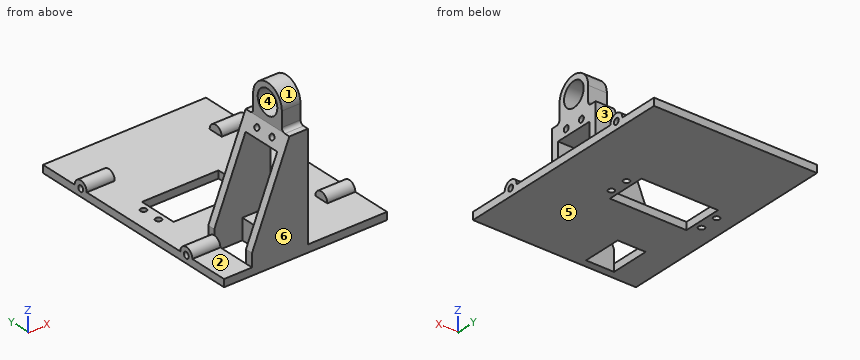
Autodesk Inventor part; units mm, degrees
ref_plane "YZ Plane" through (0, 0, 0) normal (1, 0, 0) x (0, 1, 0)
ref_plane "XZ Plane" through (0, 0, 0) normal (0, 1, 0) x (-1, 0, 0)
ref_plane "XY Plane" through (0, 0, 0) normal (0, 0, 1) x (1, 0, 0)
sketch "Sketch1" plane through (0, 0, 0) normal (0, 0, 1) x (1, 0, 0)
  line L0 (-30.65, -10.5) -> (10.35, -10.5)
  line L1 (10.35, -10.5) -> (10.35, 10.5)
  line L2 (10.35, 10.5) -> (-30.65, 10.5)
  line L3 (-30.65, 10.5) -> (-30.65, -10.5)
  line L4 (-30.65, -10.5) -> (10.35, 10.5) construction
  line L5 (10.35, -10.5) -> (-30.65, 10.5) construction
  line L6 (-43.65, -60) -> (43.65, -60)
  line L7 (43.65, -60) -> (43.65, 60)
  line L8 (43.65, 60) -> (-43.65, 60)
  line L9 (-43.65, 60) -> (-43.65, -60)
  line L10 (-43.65, -60) -> (43.65, 60) construction
  line L11 (43.65, -60) -> (-43.65, 60) construction
  point P0 (-10.15, 0)
  point P1 (0, 0)
  point P2 (-10.15, 0)
  point P3 (0, 0)
  dimension "d0" = 41
  dimension "d1" = 21
  dimension "d2" = 87.3
  dimension "d3" = 120
  dimension "d4" = 10.15
extrude "Extrusion1" add sketch "Sketch1" along normal mid plane 4
sketch "Sketch2" plane through (0, 0, 2) normal (0, 0, 1) x (1, 0, 0)
  line L0 (14, -5) -> (-34.3, -5) construction
  line L1 (-34.3, -5) -> (-34.3, 5) construction
  line L2 (-34.3, 5) -> (14, 5) construction
  line L3 (14, 5) -> (14, -5) construction
  line L4 (14, -5) -> (-34.3, 5) construction
  line L5 (-34.3, -5) -> (14, 5) construction
  point P0 (0, 0)
  point P1 (-10.15, 0)
  point P2 (-10.15, 0)
  dimension "d7" = 48.3
  dimension "d8" = 10
  dimension "d9" = 14
hole "Hole1" at (-34.3, 5, 2) at (-34.3, -5, 2) at (14, -5, 2) at (14, 5, 2) direction (0, 0, -1) diameter 3.242 end through all
sketch "Sketch3" plane through (43.65, -60, 2) normal (1, 0, 0) x (0, 0, -1)
  line L0 (4, 120) -> (0, 120)
  line L1 (0, 0) -> (0, 120)
  line L2 (4, 0) -> (0, 0)
  line L3 (4, 120) -> (4, 0)
  line L4 (0, 0) -> (0, 120)
  arc A0 (0, 29) -> (0, 21) centre (0, 25) ccw
  arc A1 (0, 99) -> (0, 91) centre (0, 95) ccw
  line L5 (0, 95) -> (0, 25) construction
  point P0 (2, 60)
  point P1 (0, 60)
  dimension "d17" = 70
extrude "Extrusion2" add sketch "Sketch3" against normal blind 15 contours L1 A1 | A0 L1
sketch "Sketch4" plane through (43.65, -60, -2) normal (1, 0, 0) x (0, 0, -1)
  line L0 (0, 120) -> (-4, 120)
  line L1 (-4, 99) -> (-4, 120)
  arc A0 (-4, 99) -> (-4, 91) centre (-4, 95) ccw
  line L2 (-4, 29) -> (-4, 91)
  arc A1 (-4, 29) -> (-4, 21) centre (-4, 25) ccw
  line L3 (-4, 0) -> (-4, 21)
  line L4 (0, 0) -> (-4, 0)
  line L5 (0, 120) -> (0, 0)
  point P0 (-2, 60)
hole "Hole2" at (43.65, 35, 2) at (43.65, -35, 2) direction (-1, 0, 0) diameter 3.242 depth 11.8 tip angle 118
mirror "Mirror1" about plane through (0, 0, 0) normal (1, 0, 0) of "Extrusion2", "Hole2"
sketch "Sketch5" plane through (0, 0, 2) normal (0, 0, 1) x (1, 0, 0)
  circle A0 centre (14, -5) radius 1.621
  circle A1 centre (-34.3, 5) radius 1.621
  circle A2 centre (-34.3, -5) radius 1.621
  circle A3 centre (14, 5) radius 1.621
  line L0 (-30.65, -10.5) -> (-30.65, 10.5)
  line L1 (-30.65, 10.5) -> (10.35, 10.5)
  line L2 (10.35, 10.5) -> (10.35, -10.5)
  line L3 (10.35, -10.5) -> (-30.65, -10.5)
  line L4 (-43.65, -31) -> (-28.65, -31)
  line L5 (-28.65, -31) -> (-28.65, -39)
  line L6 (-28.65, -39) -> (-43.65, -39)
  line L7 (-43.65, -39) -> (-43.65, -60)
  line L8 (-43.65, -60) -> (43.65, -60)
  line L9 (43.65, -60) -> (43.65, -39)
  line L10 (43.65, -39) -> (28.65, -39)
  line L11 (28.65, -39) -> (28.65, -31)
  line L12 (28.65, -31) -> (43.65, -31)
  line L13 (43.65, -31) -> (43.65, 31)
  line L14 (43.65, 31) -> (28.65, 31)
  line L15 (28.65, 31) -> (28.65, 39)
  line L16 (28.65, 39) -> (43.65, 39)
  line L17 (43.65, 39) -> (43.65, 60)
  line L18 (43.65, 60) -> (-43.65, 60)
  line L19 (-43.65, 60) -> (-43.65, 39)
  line L20 (-43.65, 39) -> (-28.65, 39)
  line L21 (-28.65, 39) -> (-28.65, 31)
  line L22 (-28.65, 31) -> (-43.65, 31)
  line L23 (-43.65, 31) -> (-43.65, -31)
  line L24 (-28.65, -35) -> (1.35, -35)
  line L25 (1.35, -35) -> (1.35, -56)
  line L26 (1.35, -56) -> (-28.65, -56)
  line L27 (-28.65, -56) -> (-28.65, -35)
  line L28 (-28.65, -31) -> (-28.65, -39)
  line L29 (10.35, 10.5) -> (10.35, -10.5)
  point P0 (0, 0)
  dimension "d27" = 45
  dimension "d28" = 4
extrude "Extrusion3" add sketch "Sketch5" along normal blind 7 contours L24 L25 L26 L27 L5
sketch "Sketch6" plane through (1.35, -56, 2) normal (1, 0, 0) x (0, 0, -1)
  line L0 (0, 21) -> (0, 0)
  line L1 (0, 21) -> (-7, 21)
  line L2 (-7, 0) -> (-7, 21)
  line L3 (0, 0) -> (-7, 0)
  line L4 (-56, -4) -> (0, -4)
  line L5 (0, -4) -> (0, 25)
  line L6 (0, 25) -> (-56, 25)
  line L7 (-56, 25) -> (-56, -4)
  line L8 (-7, 0) -> (-48, 0)
  line L9 (-48, 0) -> (-48, 21)
  line L10 (-48, 21) -> (-7, 21)
  line L11 (-7, 21) -> (-7, 0)
  line L12 (0, 25) -> (0, 87)
  line L13 (0, -4) -> (4, -4)
  point P0 (2, 56)
  point P1 (0, 10.5)
  dimension "d31" = 41
  dimension "d32" = 8
extrude "Extrusion4" add sketch "Sketch6" against normal up to surface (30 mm away) contours L0 L3 L2 L1 | L1 L10 L9 L8 L3 L5 L4 L7 L6
sketch "Sketch8" plane through (1.35, -60, 58) normal (1, 0, 0) x (0, 0, -1)
  line L0 (56, 29) -> (56, 0)
  line L1 (4.35, 9.5) -> (52.65, 9.5) construction
  line L2 (52.65, 9.5) -> (52.65, 19.5) construction
  line L3 (52.65, 19.5) -> (4.35, 19.5) construction
  line L4 (4.35, 19.5) -> (4.35, 9.5) construction
  line L5 (56, 29) -> (0, 29)
  line L6 (0, 29) -> (0, 0)
  line L7 (0, 0) -> (56, 0)
  point P0 (58, 60)
  point P1 (4.35, 14.5)
  point P2 (8, 14.5)
  point P3 (28.5, 19.5)
  point P4 (28.5, 25)
  dimension "d38" = 48.3
  dimension "d39" = 10
hole "Hole3" at (1.35, -50.5, 53.65) at (1.35, -40.5, 53.65) at (1.35, -40.5, 5.35) at (1.35, -50.5, 5.35) direction (-1, 0, 0) diameter 3.242 depth 11.8 tip angle 118
sketch "Sketch9" plane through (-43.65, -60, -2) normal (0, -1, 0) x (1, 0, 0)
  line L0 (87.3, 0) -> (87.3, 4)
  line L1 (45, 4) -> (87.3, 4)
  line L2 (45, 60) -> (45, 4)
  line L3 (45, 60) -> (15, 60)
  line L4 (15, 60) -> (15, 4)
  line L5 (0, 4) -> (15, 4)
  line L6 (0, 4) -> (0, 0)
  line L7 (87.3, 0) -> (0, 0)
  line L8 (15, 11) -> (45, 11)
  line L9 (15, 11) -> (35, 60)
  point P0 (43.65, 2)
  dimension "d47" = 10
extrude "Extrusion6" cut sketch "Sketch9" against normal through all contours L4 L3 L9
sketch "Sketch10" plane through (1.35, -60, 58) normal (1, 0, 0) x (0, 0, -1)
  circle A0 centre (52.65, 19.5) radius 1.621
  circle A1 centre (4.35, 9.5) radius 1.621
  circle A2 centre (4.35, 19.5) radius 1.621
  circle A3 centre (52.65, 9.5) radius 1.621
  line L0 (56, 29) -> (56, 0)
  line L1 (56, 29) -> (0, 29)
  line L2 (0, 29) -> (0, 0)
  line L3 (0, 0) -> (56, 0)
  line L4 (49, 4) -> (8, 4)
  line L5 (8, 4) -> (8, 25)
  line L6 (8, 25) -> (49, 25)
  line L7 (49, 4) -> (49, 25)
  circle A4 centre (-10, 14.5) radius 6.5
  arc A5 (0, 3) -> (-2, 5) centre (-2, 3) ccw
  line L8 (0, 29) -> (0, 0)
  arc A6 (-2, 24) -> (0, 26) centre (-2, 26) ccw
  line L9 (-2, 5) -> (-10, 5)
  arc A7 (-10, 24) -> (-10, 5) centre (-10, 14.5) ccw
  line L10 (-10, 24) -> (-2, 24)
  point P0 (58, 60)
  point P1 (0, 14.5)
  dimension "d50" = 13
  dimension "d51" = 10
  dimension "d52" = 3
  dimension "d53" = 2
extrude "Extrusion7" add sketch "Sketch10" against normal blind 10 contours L2 A5 L9 A7 L10 A6
sketch "Sketch11" plane through (0, 0, 9) normal (0, 0, 1) x (1, 0, 0)
  line L0 (1.35, -35) -> (-28.65, -35)
  line L1 (-28.65, -35) -> (-28.65, -56)
  line L2 (-28.65, -56) -> (1.35, -56)
  line L3 (1.35, -56) -> (1.35, -35)
  line L4 (1.35, -35) -> (-28.65, -35)
  line L5 (-28.65, -56) -> (-13.65, -56)
  line L6 (-13.65, -56) -> (-13.65, -35)
  line L7 (-13.65, -35) -> (-28.65, -35)
  line L8 (-28.65, -35) -> (-28.65, -56)
  point P0 (0, 0)
  dimension "d56" = 15
extrude "Extrusion8" cut sketch "Sketch11" against normal through all contours L6 L2 L1 L0
properties part number "Ground_Tracker_ServoMount" material "ABS Plastic"
Can you work these out from the model? Positions are in its coordinate system, mm. Face numbers are marked on the shaded views. A direction names the side the tool comes from. Coordinates: 2 decimals unless noted, no trailing zeros. Write each loop counter-clockwise with the first axis right and the second up, starting at its lowest first coordinate (ties: lowest second). Pieces come first, ordered by that corner, then holes. Notation, with made-up numbers: (72, 68.25) -> (117, 68.25) arc R20 cw to (117, 102.25) -> close; hole circle Ø3 at (56, 55). An arc over 180 degrees is marked (long way). Answer as CSV lines item,"result".
1) On a 3-axis mill with a long thin cutter (end or side, diameter ignored), from which of +Z, -Z, +X, -X, +Y, -Y can I reach the whole of each face in a straight line? I mean the marked faces 1, 2 and 3. Say none if no direction works.
Check result:
face 1,"+Z, +X, -X"
face 2,"+Z, -X, -Y"
face 3,"+Z, +X, -X, +Y"
2) If I drill on line 1 (X direction, y = -5, z = 0); line 2 (Y direction, x = -2.5, z = 53.65); line 3 (Y direction, x = 14, z = 0), over which ranges is the centre line in solid material (lowest first)? Write a range as from..to.
Check result:
line 1,"-43.65..-35.92, -32.68..-30.65, 10.35..12.38, 15.62..43.65"
line 2,"-60..-52.12, -48.88..-42.12, -38.88..-31"
line 3,"-60..-6.62, -3.38..3.38, 6.62..60"
3) Will these pins go through, and if not, where does the flat tip stop? P1, Ø12, axis at x = 21.5, y = 45.5, coming from the +Z side; P2, Ø12, axis at x = 6.5, z = 18, coming from the +Y side; P3, Ø2.5, axis at x = -4.5, y = -58, coming from the +Z side.
Check result:
P1,"z = 2"
P2,"y = -31"
P3,"z = 58.02"
4) If we section it at B-B on y = -5: Please give me the cut outline in (x, z), then the cut area to 3 significant figures.
Check result:
outline,"(-43.65, -2) -> (-35.92, -2) -> (-35.92, 2) -> (-43.65, 2) -> close; (-32.68, -2) -> (-30.65, -2) -> (-30.65, 2) -> (-32.68, 2) -> close; (10.35, -2) -> (12.38, -2) -> (12.38, 2) -> (10.35, 2) -> close; (15.62, -2) -> (43.65, -2) -> (43.65, 2) -> (15.62, 2) -> close"
area,"159 mm²"
5) If we section it at A-A on x = -7: Please give me the cut outline in (y, z), then the cut area to 3 significant figures.
Check result:
outline,"(-60, -2) -> (-10.5, -2) -> (-10.5, 2) -> (-31, 2) -> (-31, 58) -> (-34, 58) arc R2 cw to (-36, 60) -> (-36, 68) arc R9.5 ccw to (-55, 68) -> (-55, 60) arc R2 cw to (-57, 58) -> (-60, 58) -> close; (10.5, -2) -> (60, -2) -> (60, 2) -> (10.5, 2) -> close; hole (-56, 9) -> (-35, 9) -> (-35, 50) -> (-56, 50) -> close; hole circle Ø3.24 at (-50.5, 5.35); hole circle Ø3.24 at (-50.5, 53.65); hole circle Ø13 at (-45.5, 68); hole circle Ø3.24 at (-40.5, 5.35); hole circle Ø3.24 at (-40.5, 53.65)"
area,"1,330 mm²"
6) If we section it at C-C on x = 34.5: Please give me the cut outline in (y, z), then the cut area to 3 significant figures.
Check result:
outline,"(-60, -2) -> (60, -2) -> (60, 2) -> (39, 2) arc R4 ccw to (31, 2) -> (-31, 2) arc R4 ccw to (-39, 2) -> (-60, 2) -> close; hole circle Ø3.24 at (-35, 2); hole circle Ø3.24 at (35, 2)"
area,"514 mm²"
7) If we section it at D-D on z = 16.5: Please give me the cut outline in (x, y), then the cut area to 3 significant figures.
Check result:
outline,"(-25.59, -60) -> (1.35, -60) -> (1.35, -56) -> (-25.59, -56) -> close; (-25.59, -35) -> (1.35, -35) -> (1.35, -31) -> (-25.59, -31) -> close"
area,"216 mm²"
8) If we mould it in two halves opening along Y, with no side actions, what happens to the marked faces 4, 5 and 6? For each: +Y half, -Y half, draft (parallel to the pull), parting line (faces both ways), or undercut.
Check result:
face 4,"undercut"
face 5,"draft"
face 6,"-Y half"
